from build123d import *

# Parameters (mm, degrees)
SKETCH1_W           = 40
SKETCH1_H           = 30
BOSS_EXTRUDE1_DEPTH = 12
SKETCH2_W           = 25
SKETCH2_H           = 12
CUT_EXTRUDE1_DEPTH  = 12
SKETCH3_R           = 4
CUT_EXTRUDE2_DEPTH  = 100
FILLET1_R           = 5
SKETCH4_R           = 4
CUT_EXTRUDE3_DEPTH  = 12.5
SKETCH6_W           = 44.346855167
SKETCH6_H           = 29.153227126
CUT_EXTRUDE4_DEPTH  = 100
SKETCH7_W           = 40
SKETCH7_H           = 6
BOSS_EXTRUDE2_DEPTH = 20
SKETCH8_W           = 5
SKETCH8_H           = 20
SKETCH8_H_2         = 10
BOSS_EXTRUDE3_DEPTH = 6
SKETCH9_R           = 3
SKETCH9_W           = 35
SKETCH9_H           = 9
CUT_EXTRUDE5_DEPTH  = 20
CHAMFER2_SIZE2      = 6
CHAMFER2_SIZE       = 8.895365811
FILLET2_R           = 5
FILLET3_R           = 3
CHAMFER3_SIZE       = 1
FILLET4_R           = 3


with BuildPart() as part:
    # Sketch1 → Boss-Extrude1 (new body)
    with BuildSketch(Plane(origin=(0, 0, 0), x_dir=(1, 0, 0), z_dir=(0, 1, 0))):
        Rectangle(SKETCH1_W, SKETCH1_H)
    extrude(amount=BOSS_EXTRUDE1_DEPTH)

    # Sketch2 → Cut-Extrude1 (cut)
    with BuildSketch(Plane(origin=(0, 12, 0), x_dir=(1, 0, 0), z_dir=(0, 1, 0))):
        with Locations((0, 9)):
            Rectangle(SKETCH2_W, SKETCH2_H)
    extrude(amount=-CUT_EXTRUDE1_DEPTH, mode=Mode.SUBTRACT)

    # Sketch3 → Cut-Extrude2 (cut)
    with BuildSketch(Plane(origin=(20, 0, 0), x_dir=(0, 0, -1), z_dir=(1, 0, 0))):
        with Locations((9, 6)):
            Circle(SKETCH3_R)
    extrude(amount=-CUT_EXTRUDE2_DEPTH, mode=Mode.SUBTRACT)

    # Fillet1
    fillet1_edges = [part.edges().sort_by_distance(p)[0] for p in [
        (-16.25, 0, -15),
        (-16.25, 12, -15),
        (16.25, 0, -15),
        (16.25, 12, -15),
    ]]
    fillet(fillet1_edges, radius=FILLET1_R)

    # Sketch4 → Cut-Extrude3 (cut)
    with BuildSketch(Plane.XY.offset(15)):
        with Locations((-12.5, 6)):
            Circle(SKETCH4_R)
        with Locations((12.5, 6)):
            Circle(SKETCH4_R)
    extrude(amount=-CUT_EXTRUDE3_DEPTH, mode=Mode.SUBTRACT)

    # Sketch6 → Cut-Extrude4 (cut)
    with BuildSketch(Plane(origin=(0, 12, 0), x_dir=(1, 0, 0), z_dir=(0, 1, 0))):
        with Locations((2.173427584, 17.576613563)):
            Rectangle(SKETCH6_W, SKETCH6_H)
    extrude(amount=-CUT_EXTRUDE4_DEPTH, mode=Mode.SUBTRACT)

    # Sketch7 → Boss-Extrude2 (add)
    with BuildSketch(Plane(origin=(0, 0, -3), x_dir=(-1, 0, 0), z_dir=(0, 0, -1))):
        with Locations((0, 3)):
            Rectangle(SKETCH7_W, SKETCH7_H)
    extrude(amount=BOSS_EXTRUDE2_DEPTH)

    # Sketch8 → Boss-Extrude3 (add)
    with BuildSketch(Plane(origin=(0, 6, 0), x_dir=(1, 0, 0), z_dir=(0, 1, 0))):
        Polygon((15, 23), (20, 23), (20, 48.649342911), (15, 48.649342911), (15, 38.649342911), align=None)
        with Locations((17.5, 13)):
            Rectangle(SKETCH8_W, SKETCH8_H)
        with Locations((12.5, 43.649342911)):
            Rectangle(SKETCH8_W, SKETCH8_H_2)
    extrude(amount=BOSS_EXTRUDE3_DEPTH)

    # Sketch9 → Cut-Extrude5 (cut)
    with BuildSketch(Plane(origin=(0, 6, 0), x_dir=(1, 0, 0), z_dir=(0, 1, 0))):
        with Locations(Location((-12, 9, 0), (0, 0, 270))):
            Circle(SKETCH9_R)
        with Locations((-2.5, 18.5)):
            Rectangle(SKETCH9_W, SKETCH9_H)
    extrude(amount=-CUT_EXTRUDE5_DEPTH, mode=Mode.SUBTRACT)

    # Chamfer2
    chamfer2_edges = [part.edges().sort_by_distance(p)[0] for p in [
        (17.5, 0, -23),
    ]]
    chamfer2_side = [part.faces().sort_by_distance(p)[0] for p in [
        (17.5, 0, -22.88),
    ]]
    chamfer(chamfer2_edges, length=CHAMFER2_SIZE - 0.0001, length2=CHAMFER2_SIZE2 - 0.0001, reference=chamfer2_side[0])  # a hair under: the kernel refuses the full size

    # Fillet2
    fillet2_edges = [part.edges().sort_by_distance(p)[0] for p in [
        (-20, 3, -14),
        (15, 3, -14),
    ]]
    fillet(fillet2_edges, radius=FILLET2_R)

    # Fillet3
    fillet3_edges = [part.edges().sort_by_distance(p)[0] for p in [
        (-2.5, 6, -3),
        (15, 6, -11),
        (15, 9, -3),
    ]]
    fillet(fillet3_edges, radius=FILLET3_R - 0.0001)  # a hair under: the kernel refuses the full size

    # Chamfer3
    chamfer3_edges = [part.edges().sort_by_distance(p)[0] for p in [
        (15, 12, -48.649342911),
        (10, 12, -43.649342911),
        (15, 12, -22.324621456),
        (12.5, 12, -38.649342911),
        (0, 12, 15),
        (14.121349633, 12, -3.878650367),
        (-3.99995, 12, -3),
        (20, 12, -16.824671456),
        (-20, 12, 6),
    ]]
    chamfer(chamfer3_edges, length=CHAMFER3_SIZE)

    # Fillet4
    fillet4_edges = [part.edges().sort_by_distance(p)[0] for p in [
        (15, 8.5, -38.649342911),
    ]]
    fillet(fillet4_edges, radius=FILLET4_R)


solid = part.part
Read the model definition and answer for the solid it produces. Units are mm, in the model's axes. A direction names the side the tool comes from. Give positions to 0.01 mm unless a question says otherwise; leave off trailing zeros. Write each loop counter-clockwise with the first axis right and the second up, starting at its lowest first coordinate (ties: lowest second). Pieces come first, ordered by that corner, then holes. Notation, with made-up numbers: M 36.25,-6 L 94.25,-6 A16 ccw 94.25,8 Z; hole C 30,7 d3. An arc over 180 degrees is marked long. One line per item, written item: value. Start each with the question number.
(1) Determine the mould class of faces 1 (the cylindrical face through (14.1, 6.86, -10.96)), 2 (the cylindrical face through (9.3, 3.6, 8.8)), 3 (the flat face through (-13, 6, 2.5)) for opening direction Z: pulls with the +Z half, pulls with the -Z half, needs draft (parallel to the pull), parting line crosses it, or undercut.
(2) Find the intervals of material crossed by line 1 (X direction, y = 6.25, z = 10); line 2 (Z direction, x = 12, y = 9.75); line 3 (Y direction, x = 12.5, z = 7.25), in increasing order.
(3) Find section A-A (z = 8). Determine the outline of the cut face in (x, y).
(4) Find section D-D (y = 4.75). Determine the outline of the cut face in (x, z).
(5) A tool of negligible diameter and unlimited length cuts with its end or side. For faces 4 (the flat face through (-3, 3, -14)), 5 (the flat face through (12, 6, 2.5)), 6 (the cylindrical face through (14, 4, -16)), from which of +Z, -Z, +X, -X, +Y, -Y can it reach the whole face along a straight path? Write none if from no direction.
(6) Find section C-C (z = -29.5). Determine the outline of the cut face in (x, y).
(7) Find section B-B (x = -13). Determine the outline of the cut face in (y, z), plus the area to 3 significant figures.
(8) Flat-ended cylindrical pins translate along their axes: pin 1 Ø1.5 at (y, z) = (8, -42.5) entering from -X; pin 2 Ø5 at (x, y) = (-15, 10) entering from -Z; pin 3 Ø1.5 at (y, z) = (10.5, -32.5) entering from -X. Find the tip coordinate at first contact, or state that the pin passes through.
Results below:
1. face 1: undercut
1. face 2: needs draft
1. face 3: pulls with the +Z half
2. line 1: x = -20 to -16.49, -8.51 to 8.51, 16.49 to 20
2. line 2: z = -48.65 to -38.65, -3 to 2.5
2. line 3: y = 0 to 2, 10 to 12
3. outline: M -20,0 L 20,0 L 20,11 L 19,12 L -19,12 L -20,11 Z; hole C -12.5,6 d8; hole C 12.5,6 d8
4. outline: M -20,-9 A5 ccw -15,-14 L 10,-14 A5 cw 15,-19 L 15,-21.15 L 20,-21.15 L 20,15 L 16.3,15 L 16.3,2.5 L 8.7,2.5 L 8.7,15 L -8.7,15 L -8.7,2.5 L -16.3,2.5 L -16.3,15 L -20,15 Z; hole C -12,-9 d6
5. face 4: -Z, -X, +Y, -Y
5. face 5: +Z
5. face 6: -X, +Y, -Y
6. outline: M 15,6 L 20,6 L 20,11 L 19,12 L 16,12 L 15,11 Z
7. outline: M 0,-14 L 6,-14 L 6,-11.83 L 0,-11.83 Z; M 0,-6.17 L 6,-6.17 L 6,-6 A3 cw 9,-3 L 11,-3 L 12,-2 L 12,14 L 11,15 L 9.97,15 L 9.97,2.5 L 2.03,2.5 L 2.03,15 L 0,15 Z
7. area: 150 mm^2
8. pin 1: stops at x = 10
8. pin 2: stops at z = -3.4
8. pin 3: stops at x = 15
